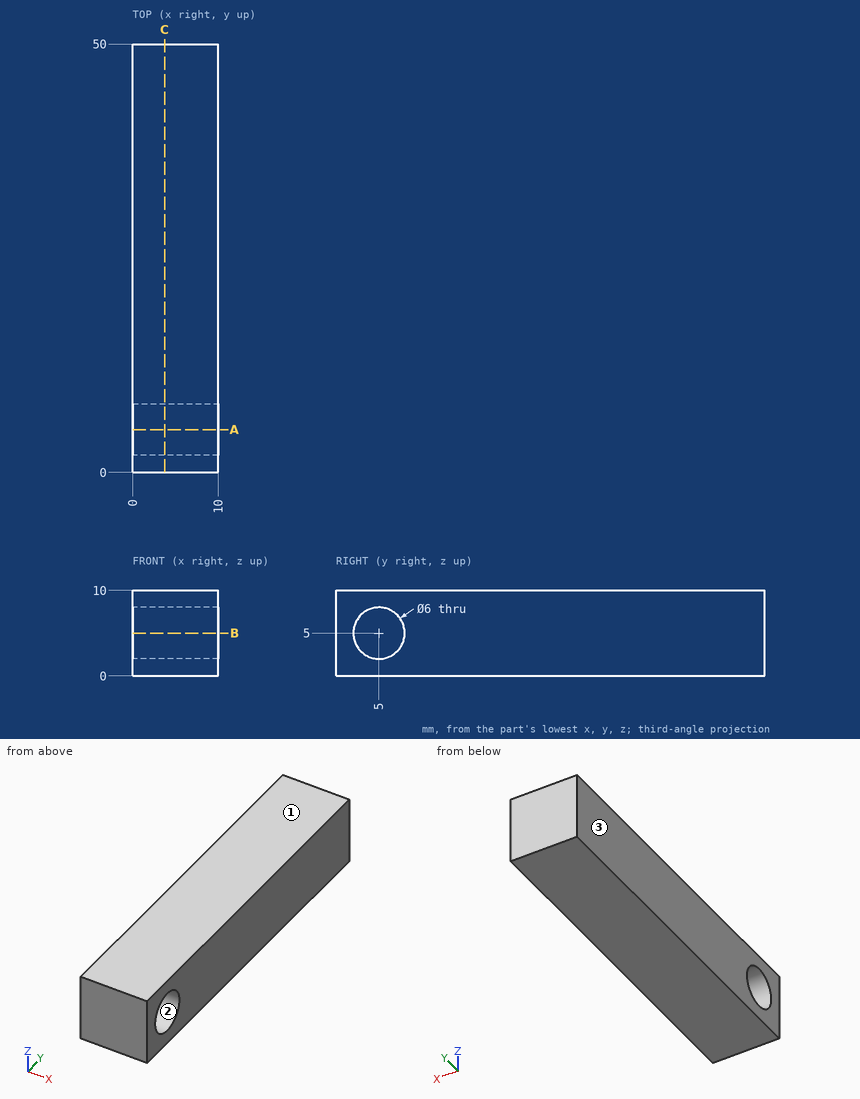
Job drawing, mm, ordinate dimensions from the low corner. One solid piece. Give positions to 0.01 mm unless a question says otherwise; leave off trailing zeros. Loops run counter-clockwise (first coordinate to the right, second up) from the corner with the lowest first, then second, coordinate; pieces in that order, holes last. Notation, with made-up numbers: (55.25, 28) - (94.25, 28) arc R25 ccw to (94.25, 42) - close; hole circle Ø11 at (-31.75, 42). An arc over 180 degrees is marked (long way). Use one line per item in the form item = value.
(1) Cut at C-C (x = 3.75). Give the cut face in (y, z), then the cut area to 3 significant figures.
Determined:
outline = (0, 0) - (50, 0) - (50, 10) - (0, 10) - close; hole circle Ø6 at (5, 5)
area = 472 mm^2
(2) Cut at A-A (y = 5). Give the cut face in (x, z), then the cut area to 3 significant figures.
Determined:
outline = (0, 0) - (10, 0) - (10, 2) - (0, 2) - close; (0, 8) - (10, 8) - (10, 10) - (0, 10) - close
area = 40.0 mm^2
(3) Cut at B-B (z = 5). Give the cut face in (x, y), then the cut area to 3 significant figures.
Determined:
outline = (0, 0) - (10, 0) - (10, 2) - (0, 2) - close; (0, 8) - (10, 8) - (10, 50) - (0, 50) - close
area = 440 mm^2
(4) Drill centre lines: L1, parallel to Z at x = 8, y = 5; L2, parallel to Y at x = 2.5, z = 7; L3, parallel to Y at x = 6, z = 7.5. Where is each one in solid material? Low to high.
Determined:
L1 = 0 to 2, 8 to 10
L2 = 0 to 2.76, 7.24 to 50
L3 = 0 to 3.34, 6.66 to 50
(5) Pull direction Z, two halves, no side cores. Call the marked faces 1, 2 and 3: pulls with the +Z half, pulls with the -Z half, needs draft (parallel to the pull), parting line crosses it, or undercut.
Determined:
face_1 = pulls with the +Z half
face_2 = undercut
face_3 = needs draft
